Build history of the part. All positions in model axes, mm. A direction names the side the tool comes from. Give positions to 0.01 mm unless a question says otherwise; leave off trailing zeros. Order: outer loops, then holes, each group sorted by start corner. A loop starts at its lowest first (then second) coordinate and runs counter-clockwise, first axis right, second up. Notation, with made-up numbers: (21.25, 85.5) - (67.25, 85.5) arc R12 ccw to (67.25, 101.5) - close; hole circle Ø11 at (-31, -5). An arc over 180 degrees is marked (long way). Use a Markdown table: item, result. Add a question column.
(1) Flat gauge pins, fed straight in: pin 1 (1 mm diameter, centred on y = 22.5, z = 2, fed in from +X) (3 decimals); pin 2 (6 mm diameter, centred on x = 5.5, y = 19.5, fed in from +Z); pin 3 (1 mm diameter, centred on y = 12.5, z = 1, fed in from -X). Where does each tip first touch, or does it go through?
(2) Wall check: line 1 (Y direction, x = -5, z = 2.15); line 2 (X direction, y = 12.5, z = 1.25) (3 decimals); line 3 (X direction, y = 11, z = 1.45). Give the ranges that are in metal, low to high.
(3) Mould opens along Y. For faces 3 (the face through (0, -25.4, 2)), 4 (the face through (-1, 50.8, 2)), 5 (the face through (39.71, -0.711, 1.565)) say: +Y half, -Y half, draft (parallel to the pull), parting line (faces both ways), or undercut.
(4) Slice it at C-C (z = 1.6). Write the cut outline in (x, y).
(5) Slice it at B-B (x = -15). Write the cut outline in (y, z) (3 decimals), then the cut area to 3 significant figures.
(6) Which spindle directions (+Z, -Z, +X, -X, +Y, -Y) get a long thin tool onto all of the face, cutting with end or side? Do faces 1 (the face through (19.05, 0, 2)), 2 (the face through (-25, 1, 0)). Say none if no direction does.
from build123d import *

# Parameters (mm, degrees)
F0_W     = 82.55
F0_H     = 101.6
F1_DEPTH = 3.175
F2_SIZE  = 3.17499
F3_W     = 38.1
F3_H     = 50.8
F4_DEPTH = 3.175
F5_SIZE  = 3.17499


# Not quite as in the source:
# - a fillet or chamfer is up to 0.001 mm smaller than in the source, because OpenCascade refuses the exact size


with BuildPart() as f1:
    # F0 (on Top) → F1 (new body)
    with BuildSketch(Plane.XY):
        Rectangle(F0_W, F0_H)
    extrude(amount=F1_DEPTH)

    # F2 (size 3.175 in the source; OpenCascade refuses exactly that, so slightly less here)
    f2_edges = [f1.edges().sort_by_distance(p)[0] for p in [
        (-41.275, 0, 0),
    ]]
    chamfer(f2_edges, length=F2_SIZE)

    # F3 (on face) → F4 (cut)
    with BuildSketch(Plane(origin=(0, 0, 0), x_dir=(1, 0, 0), z_dir=(0, 0, -1))):
        Rectangle(F3_W, F3_H)
    extrude(amount=-F4_DEPTH, mode=Mode.SUBTRACT)

    # F5 (size 3.175 in the source; OpenCascade refuses exactly that, so slightly less here)
    f5_edges = [f1.edges().sort_by_distance(p)[0] for p in [
        (41.275, 0, 3.175),
    ]]
    chamfer(f5_edges, length=F5_SIZE)


solid = f1.part
Solution:
| question | item | result |
|---|---|---|
| 1 | pin 1 | x = 39.775 |
| 1 | pin 2 | through |
| 1 | pin 3 | x = -39.6 |
| 2 | line 1 | -50.8 to -25.4, 25.4 to 50.8 |
| 2 | line 2 | -39.35 to -19.05, 19.05 to 40.025 |
| 2 | line 3 | -39.55 to -19.05, 19.05 to 39.83 |
| 3 | face 3 | undercut |
| 3 | face 4 | +Y half |
| 3 | face 5 | draft |
| 4 | outline | (-39.7, -50.8) - (39.68, -50.8) - (39.68, 50.8) - (-39.7, 50.8) - close; hole (-19.05, -25.4) - (19.05, -25.4) - (19.05, 25.4) - (-19.05, 25.4) - close |
| 5 | outline | (-50.8, 0) - (-25.4, 0) - (-25.4, 3.175) - (-50.8, 3.175) - close; (25.4, 0) - (50.8, 0) - (50.8, 3.175) - (25.4, 3.175) - close |
| 5 | area | 161 mm2 |
| 6 | face 1 | +Z, -Z |
| 6 | face 2 | -Z, +X, -X, +Y, -Y |
